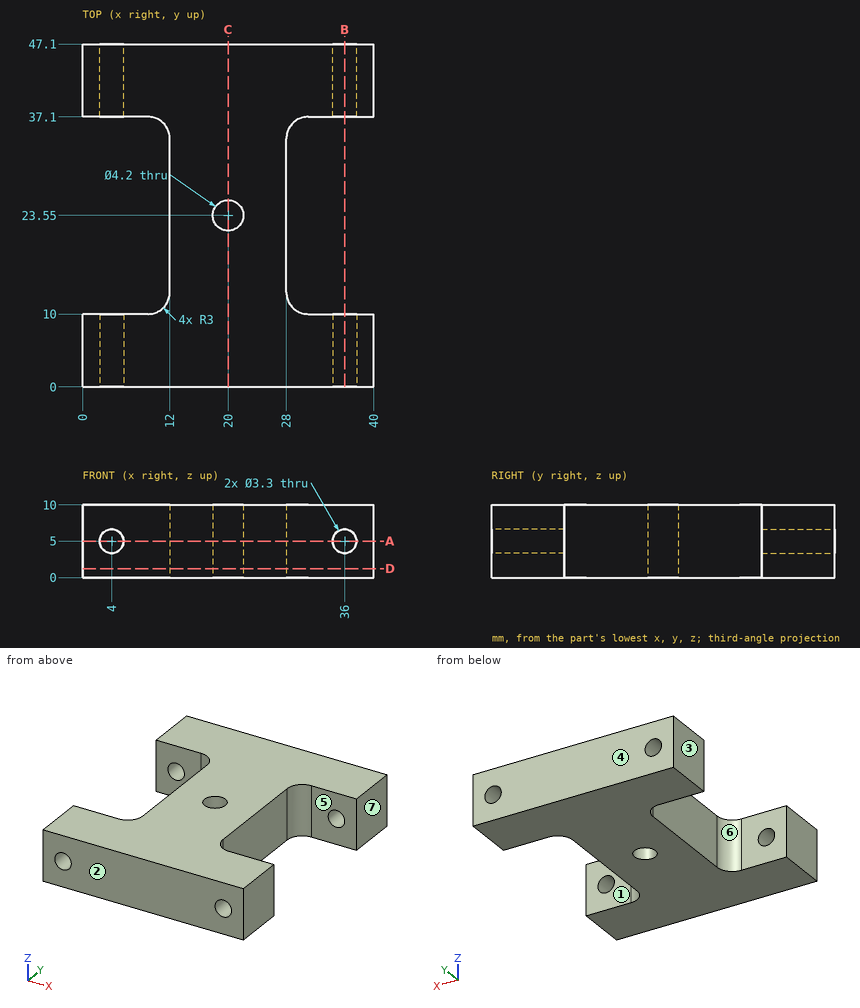
Verification items for this drawing (mm, ordinates from the low corner). A direction names the side the tool comes from. Round coordinates to 2 decimals unless told otherwise and drop trailing zeros. Loops run counter-clockwise (first coordinate to the right, second up) from the corner with the lowest first, then second, coordinate; pieces in that order, holes last. Notation, with made-up numbers: (-33.75, 1.5) -> (-21.75, 1.5) arc R32 ccw to (-21.75, 27.5) -> close; hole circle Ø5 at (-2, 78.25). An arc over 180 degrees is marked (long way). Write item = value, one per line. Start each with the question number.
1) Thickness scan on probe 1 along X at (y, z) = (44, 5); probe 2 along Y at (x, z) = (5.5, 6); probe 3 along Y at (x, z) = (20, 6). Record the ranges inside material, lowest first.
2) Set-up check for the marked faces 5, 6 and 7: record each of +Z, -Z, +X, -X, +Y, -Y from which the full face is reachable in a straight line by a thin tool's end or side.
3) Sectioned sample at C-C, the plane x = 20. Record the cut outline in (y, z).
4) Sectioned sample at D-D, the plane z = 1.25. Record the cut outline in (x, y).
5) Release check for a two-part mould opening along Y. For the marked faces 1, 2, 3 and 4 record: released by +Y, released by -Y, zero draft, split by the parting line, or undercut.
6) Sectioned sample at B-B, the plane x = 36. Record the cut outline in (y, z), plus the area to 3 significant figures.
7) Sectioned sample at A-A, the plane z = 5. State how many separate pieces and enclosed holes the cut face has, plus the area to 3 significant figures.
8) Gauge pin test, flat ends, axial feed: pin 1 Ø2 at (x, z) = (36, 5) entering from -Y; pin 2 Ø1.5 at (y, z) = (31, 4) entering from +X. Record the tip position at first contact, or that the pin passes through.
Results are:
q1.probe_1 = 0 to 2.35, 5.65 to 34.35, 37.65 to 40
q1.probe_2 = 0 to 10, 37.1 to 47.1
q1.probe_3 = 0 to 21.45, 25.65 to 47.1
q2.face_5 = +Z, -Z, +X
q2.face_6 = +Z, -Z, -X
q2.face_7 = +Z, -Z, +X, +Y, -Y
q3.outline = (0, 0) -> (21.45, 0) -> (21.45, 10) -> (0, 10) -> close; (25.65, 0) -> (47.1, 0) -> (47.1, 10) -> (25.65, 10) -> close
q4.outline = (0, 0) -> (40, 0) -> (40, 10) -> (31, 10) arc R3 cw to (28, 13) -> (28, 34.1) arc R3 cw to (31, 37.1) -> (40, 37.1) -> (40, 47.1) -> (0, 47.1) -> (0, 37.1) -> (9, 37.1) arc R3 cw to (12, 34.1) -> (12, 13) arc R3 cw to (9, 10) -> (0, 10) -> close; hole circle Ø4.2 at (20, 23.55)
q5.face_1 = undercut
q5.face_2 = released by -Y
q5.face_3 = zero draft
q5.face_4 = released by +Y
q6.outline = (0, 0) -> (10, 0) -> (10, 3.35) -> (0, 3.35) -> close; (0, 6.65) -> (10, 6.65) -> (10, 10) -> (0, 10) -> close; (37.1, 0) -> (47.1, 0) -> (47.1, 3.35) -> (37.1, 3.35) -> close; (37.1, 6.65) -> (47.1, 6.65) -> (47.1, 10) -> (37.1, 10) -> close
q6.area = 134 mm^2
q7.separate_pieces = 5
q7.enclosed_holes = 1
q7.area = 1,100 mm^2
q8.pin_1 = through
q8.pin_2 = 28
